For this review, take the finished solid that the model builds, in its own axes (mm). Face numbers are marked on the shaded views. A direction names the side the tool comes from. Coordinates: 2 decimals unless noted, no trailing zeros. Order: outer loops, then holes, each group sorted by start corner. A loop starts at its lowest first (then second) coordinate and runs counter-clockwise, first axis right, second up. Notation, with made-up numbers: (43.5, 4) -> (56.5, 4) arc R19 cw to (56.5, 32) -> close; hole circle Ø11 at (-39.75, 45.25). An arc over 180 degrees is marked (long way). Write item = value, one per line. Start each with the question number.
1) Wall thickness on probe 1 along X at (y, z) = (41, 22.25); probe 2 along Y at (x, z) = (220, 14.5); probe 3 along Y at (x, z) = (117, 23.5): over which ranges is each line inside the solid? List them lowest first. Write a range as [from, to].
2) Consider section D-D on z = 20.5. Give the boundary of the cut face in (x, y), and give its area (3 significant figures).
3) Draft analysis for pull direction X (two halves, no side actions). For the marked faces 3, 4, 5 and 6, state which applies: +X half, -X half, draft (parallel to the pull), parting line (faces both ways), or undercut.
4) Machinability: for the marked faces 1 and 2, which of the approach directions +Z, -Z, +X, -X, +Y, -Y give a long, thin tool a straight path to every point of the face, cutting with its end or side? Answer none if there is none.
5) Insertion check: pin 1 Ø10 at (y, z) = (102, 13) entering from +X; pin 2 Ø4 at (x, y) = (161, 43.5) entering from -Z; pin 3 Ø3 at (x, z) = (271.5, 22) entering from +Y; pin 4 Ø5 at (x, y) = (273, 86.5) entering from -Z. Each pin has a flat end and moves straight along its axis. Give the tip position at first contact, or say it passes through.
6) Consider section A-A on y = 33.5. Give the boundary of the cut face in (x, z).
7) Consider section C-C on x = 233. Give the boundary of the cut face in (y, z), and give its area (3 significant figures).
8) Consider section B-B on z = 7.75. Give the boundary of the cut face in (x, y), and give its area (3 significant figures).
Solid Edge part; units mm, degrees
sketch "Sketch1" plane through (0, 0, 0) normal (0, 0, 1) x (1, 0, 0)
  line L0 (105.1974, 149.4572) -> (268.1974, 149.4572)
  line L1 (268.1974, 149.4572) -> (268.1974, 19.4572)
  line L2 (268.1974, 19.4572) -> (105.1974, 19.4572)
  line L3 (105.1974, 19.4572) -> (105.1974, 149.4572)
  dimension "D1" = 105.1974
  dimension "D2" = 268.1974
extrude "Protrusion1" add sketch "Sketch1" along normal blind 27
sketch "Sketch2" plane through (170.1974, 84.4572, 27) normal (0, 0, 1) x (1, 0, 0)
  line L0 (-62, 62) -> (-62, -62)
  line L1 (-62, -62) -> (95, -62)
  line L2 (95, -62) -> (95, 62.14)
  line L3 (-62, 62) -> (95, 62.14)
  dimension "D1" = 62
  dimension "D2" = 95
extrude "ExtrudedCutout_1" cut sketch "Sketch2" against normal blind 23
sketch "Sketch3" plane through (170.1974, 84.5136, 4) normal (0, 0, 1) x (1, 0, 0)
  circle A0 centre (-57, -0.0564) radius 2
  circle A1 centre (-48, -0.0564) radius 2
extrude "Cutout1" cut sketch "Sketch3" against normal through all
sketch "Sketch4" plane through (186.6974, 84.4572, 0) normal (0, 0, -1) x (1, 0, 0)
  circle A0 centre (12.5, 0) radius 60
extrude "Cutout2" cut sketch "Sketch4" against normal through all
sketch "Sketch5" plane through (268.1974, 84.4572, 13.5) normal (1, 0, 0) x (0, 0, 1)
  line L0 (13.5, 0) -> (13.5, 5)
  line L1 (13.5, 5) -> (3.5, 5)
  line L2 (3.5, -5) -> (3.5, 5)
  line L3 (13.5, -5) -> (3.5, -5)
  line L4 (13.5, 0) -> (13.5, -5)
  dimension "D1" = 13.5
  dimension "D2" = 13.5
  dimension "D3" = 13.5
  dimension "D4" = 13.5
extrude "ExtrudedProtrusion_7" add sketch "Sketch5" along normal blind 10
sketch "Sketch6" plane through (273.1974, 84.4572, 17) normal (0, 0, -1) x (1, 0, 0)
  circle A0 centre (0, 0) radius 2
extrude "Cutout3" cut sketch "Sketch6" against normal through all
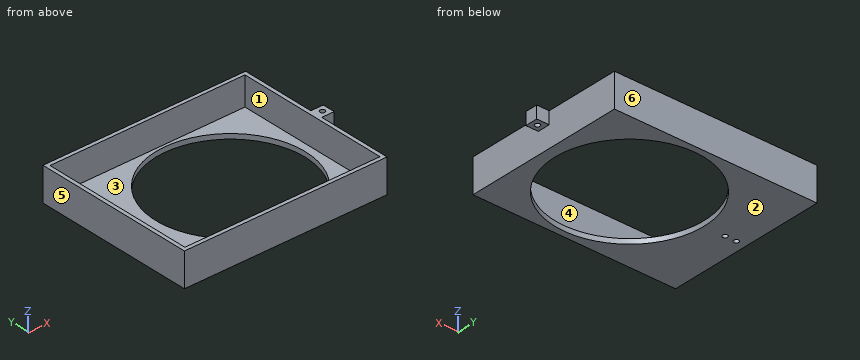
Answer sheet:
q1.probe_1 = [105.2, 108.2], [265.2, 268.2]
q1.probe_2 = [19.46, 22.46], [146.56, 149.46]
q1.probe_3 = [19.46, 22.46], [146.47, 149.46]
q2.outline = (105.2, 19.46) -> (268.2, 19.46) -> (268.2, 79.46) -> (278.2, 79.46) -> (278.2, 89.46) -> (268.2, 89.46) -> (268.2, 149.46) -> (105.2, 149.46) -> close; hole (108.2, 22.46) -> (265.2, 22.46) -> (265.2, 146.6) -> (108.2, 146.46) -> close; hole circle Ø4 at (273.2, 84.46)
q2.area = 1,800 mm2
q3.face_3 = undercut
q3.face_4 = undercut
q3.face_5 = -X half
q3.face_6 = draft
q4.face_1 = +Z
q4.face_2 = -Z, +X, -X, +Y, -Y
q5.pin_1 = 268.2
q5.pin_2 = through
q5.pin_3 = 89.46
q5.pin_4 = 17
q6.outline = (105.2, 0) -> (167.52, 0) -> (167.52, 4) -> (108.2, 4) -> (108.2, 27) -> (105.2, 27) -> close; (230.87, 0) -> (268.2, 0) -> (268.2, 27) -> (265.2, 27) -> (265.2, 4) -> (230.87, 4) -> close
q7.outline = (19.46, 0) -> (34.89, 0) -> (34.89, 4) -> (22.46, 4) -> (22.46, 27) -> (19.46, 27) -> close; (134.03, 0) -> (149.46, 0) -> (149.46, 27) -> (146.57, 27) -> (146.57, 4) -> (134.03, 4) -> close
q7.area = 259 mm2
q8.outline = (105.2, 19.46) -> (268.2, 19.46) -> (268.2, 149.46) -> (105.2, 149.46) -> close; hole (108.2, 22.46) -> (265.2, 22.46) -> (265.2, 146.6) -> (108.2, 146.46) -> close
q8.area = 1,710 mm2
